The listing builds one solid part. Answer for the finished solid, in the listing's coordinates (mm). A direction names the side the tool comes from. Round coordinates to 2 decimals unless told otherwise and drop trailing zeros. Write each loop counter-clockwise with the first axis right and the second up, starting at its lowest first coordinate (ties: lowest second). Pieces come first, ordered by that corner, then holes.
(1) Find the intervals of material crossed by probe 1 along Z at (x, y) = (26, -7.5); probe 2 along X at (y, z) = (-12, -38.5); probe 3 along X at (y, z) = (-46, -39), in increasing order.
(2) A cutting plane is placed at A-A, the plane y = -17.5. Give the vertices of the cut face in (x, z), and give its area (3 significant figures).
(3) A cutting plane is placed at B-B, the plane y = -7.5. Give the vertices of the cut face in (x, z), and give its area (3 significant figures).
(4) A cutting plane is placed at D-D, the plane y = -2.5. Give the vertices of the cut face in (x, z), and give its area (3 significant figures).
(5) For faces 1 (the face through (8, -25, -41)), 2 (the face through (-1, 0, -17)), 3 (the face through (13, -45, -5)), determine the directions among +Z, -Z, +X, -X, +Y, -Y from which every point of the face is accessible in a straight line to the end or side of a thin tool.
(6) Each of these flat-tipped pins is pushed along its axis until it touches: pin 1 Ø3.5 at (x, z) = (-1.5, -14.5) entering from -Y; pin 2 Ø3 at (x, z) = (10, -40.5) entering from +Y; pin 3 Ø2 at (x, z) = (-7, -21) entering from -Y; pin 4 Ø4.5 at (y, z) = (-7.5, -6.16) entering from -X. Where does it stop, or does it pass through?
(7) The mould has two halves that part along X. Classify faces 4 (the face through (43.88, -24.65, -53.13)), 5 (the face through (-13.6, -7.825, -30.234)), 6 (the face through (0, -20, -17)): +X half, -X half, draft (parallel to the pull), parting line (faces both ways), or undercut.
(8) A cutting plane is placed at C-C, the plane x = 9. Give the vertices of the cut face in (y, z).
from build123d import *

# Parameters (mm, degrees)
F0_W      = 75
F0_H      = 75
F1_DEPTH  = 45
F2_R      = 5
F3_R      = 12.5
F4_DEPTH  = 25
F7_DEPTH  = 25
F9_DEPTH  = 75.001
F10_DEPTH = 25
F11_R     = 2.5
F12_DEPTH = 75.001
F13_DEPTH = 25
F14_DEPTH = 20


with BuildPart() as f1:
    # F0 (on Front) → F1 (new body)
    with BuildSketch(Plane.XZ):
        with Locations((7.8840382397, -17.0557253063)):
            Rectangle(F0_W, F0_H)
    extrude(amount=F1_DEPTH)

    # F2
    f2_edges = [f1.edges().sort_by_distance(p)[0] for p in [
        (-29.615962, -22.5, 20.444275),
        (-29.615962, -22.5, -54.555725),
        (45.384038, -22.5, -54.555725),
        (45.384038, -22.5, 20.444275),
    ]]
    fillet(f2_edges, radius=F2_R)

    # F3 (on face) → F4 (cut)
    with BuildSketch(Plane.XZ.offset(45)):
        with Locations((7.8840382397, -17.0557253063)):
            Circle(F3_R)
    extrude(amount=-F4_DEPTH, mode=Mode.SUBTRACT)

    # F6 (on face) → F7 (cut)
    with BuildSketch(Plane.XZ):
        Polygon((12.8703957796, 0.5023097037), (2.8703957796, 0.4370668321), (2.8703957796, -54.635066539), (12.8703957796, -54.635066539), align=None)
    extrude(amount=F7_DEPTH, mode=Mode.SUBTRACT)

    # F8 (on face) → F9 (cut, through all)
    with BuildSketch(Plane(origin=(-29.6159617603, 0, 0), x_dir=(0, -1, 0), z_dir=(-1, 0, 0))):
        with BuildLine():
            ThreePointArc((10, -27.7557253063), (7.5, -25.2557253063), (5, -27.7557253063))
            ThreePointArc((5, -27.7557253063), (7.5, -30.2557253063), (10, -27.7557253063))
        make_face()
        with BuildLine():
            ThreePointArc((10, -6.1557253063), (7.5, -3.6557253063), (5, -6.1557253063))
            ThreePointArc((5, -6.1557253063), (7.5, -8.6557253063), (10, -6.1557253063))
        make_face()
    extrude(amount=-F9_DEPTH, mode=Mode.SUBTRACT)

    # F10 (add): a face of the model
    f10_faces = [f1.faces().sort_by_distance(p)[0] for p in [
        (44.3233780679, -45, -17.0557253063),
    ]]
    extrude(f10_faces, amount=F10_DEPTH)

    # F11 (on face) → F12 (cut, through all)
    with BuildSketch(Plane(origin=(-29.6159617603, 0, 0), x_dir=(0, -1, 0), z_dir=(-1, 0, 0))):
        with BuildLine():
            ThreePointArc((55, 10.4442746937), (54.267766953, 12.2120416467), (52.5, 12.9442746937))
            Line((52.5, 12.9442746937), (52.5, 10.4442746937))
            Line((52.5, 10.4442746937), (50, 10.4442746937))
            ThreePointArc((50, 10.4442746937), (52.5, 7.9442746937), (55, 10.4442746937))
        make_face()
        with Locations((17.5, 10.4442746937)):
            Circle(F11_R)
        with BuildLine():
            Line((52.5, 10.4442746937), (52.5, 12.9442746937))
            ThreePointArc((52.5, 12.9442746937), (50.732233047, 12.2120416467), (50, 10.4442746937))
            Line((50, 10.4442746937), (52.5, 10.4442746937))
        make_face()
    extrude(amount=-F12_DEPTH, mode=Mode.SUBTRACT)

    # F5 (on face) → F13 (cut)
    with BuildSketch(Plane.XZ.offset(45)):
        with BuildLine():
            ThreePointArc((7.8840382397, 8.1942746937), (-9.9704079852, -34.9101715312), (33.1340382397, -17.0557253063))
            ThreePointArc((33.1340382397, -17.0557253063), (25.7384844647, 0.7987209187), (7.8840382397, 8.1942746937))
        make_face()
    extrude(amount=F13_DEPTH, mode=Mode.SUBTRACT)

    # F14 (cut): a face of the model
    f14_faces = [f1.faces().sort_by_distance(p)[0] for p in [
        (44.3233780679, -70, -17.0557253063),
    ]]
    extrude(f14_faces, amount=-F14_DEPTH, mode=Mode.SUBTRACT)


solid = f1.part
Solutions:
1. probe 1: z = -54.56 to -30.26, -25.26 to -8.66, -3.66 to 20.44
1. probe 2: x = -29.62 to 2.87, 12.87 to 45.38
1. probe 3: x = -29.62 to -4.61, 20.37 to 45.38
2. outline: (-29.62, -49.56) arc R5 ccw to (-24.62, -54.56) - (2.87, -54.56) - (2.87, 0.44) - (12.87, 0.5) - (12.87, -54.56) - (40.38, -54.56) arc R5 ccw to (45.38, -49.56) - (45.38, 7.94) - (-29.62, 7.94) - close; (-29.62, 12.94) - (45.38, 12.94) - (45.38, 15.44) arc R5 ccw to (40.38, 20.44) - (-24.62, 20.44) arc R5 ccw to (-29.62, 15.44) - close
2. area: 4,680 mm2
3. outline: (-29.62, -49.56) arc R5 ccw to (-24.62, -54.56) - (2.87, -54.56) - (2.87, -30.26) - (-29.62, -30.26) - close; (-29.62, -25.26) - (2.87, -25.26) - (2.87, -8.66) - (-29.62, -8.66) - close; (-29.62, -3.66) - (2.87, -3.66) - (2.87, 0.44) - (12.87, 0.5) - (12.87, -3.66) - (45.38, -3.66) - (45.38, 15.44) arc R5 ccw to (40.38, 20.44) - (-24.62, 20.44) arc R5 ccw to (-29.62, 15.44) - close; (12.87, -54.56) - (40.38, -54.56) arc R5 ccw to (45.38, -49.56) - (45.38, -30.26) - (12.87, -30.26) - close; (12.87, -25.26) - (45.38, -25.26) - (45.38, -8.66) - (12.87, -8.66) - close
3. area: 4,400 mm2
4. outline: (-29.62, -49.56) arc R5 ccw to (-24.62, -54.56) - (2.87, -54.56) - (2.87, 0.44) - (12.87, 0.5) - (12.87, -54.56) - (40.38, -54.56) arc R5 ccw to (45.38, -49.56) - (45.38, 15.44) arc R5 ccw to (40.38, 20.44) - (-24.62, 20.44) arc R5 ccw to (-29.62, 15.44) - close
4. area: 5,050 mm2
5. face 1: -Z, +Y
5. face 2: +Z, -Z, +X, -X, +Y
5. face 3: -Y
6. pin 1: stops at y = -20
6. pin 2: stops at y = -25
6. pin 3: stops at y = -45
6. pin 4: passes through
7. face 4: +X half
7. face 5: draft
7. face 6: undercut
8. outline: (-50, -54.56) - (-25, -54.56) - (-25, -29.51) - (-45, -29.51) - (-45, -42.28) - (-50, -42.28) - close; (-50, 8.17) - (-45, 8.17) - (-45, -4.61) - (-25, -4.61) - (-25, 0.48) - (0, 0.48) - (0, 20.44) - (-50, 20.44) - close; hole circle Ø5 at (-17.5, 10.44)
